Geometry check sheet. Reference: the model listing, model coordinates, mm. Coordinates: 2 decimals unless noted, no trailing zeros. Order: outer loops, then holes, each group sorted by start corner. A loop starts at its lowest first (then second) coordinate and runs counter-clockwise, first axis right, second up. Notation, with made-up numbers: (55.25, 61.5) -> (93.25, 61.5) arc R26 ccw to (93.25, 76.5) -> close; hole circle Ø11 at (32.5, -3.5). An arc over 180 degrees is marked (long way). Answer in a Markdown table with one row per item. Add a question column.
Autodesk Inventor part; units mm, degrees
ref_plane "YZ Plane" through (0, 0, 0) normal (1, 0, 0) x (0, 1, 0)
ref_plane "XZ Plane" through (0, 0, 0) normal (0, 1, 0) x (-1, 0, 0)
ref_plane "XY Plane" through (0, 0, 0) normal (0, 0, 1) x (1, 0, 0)
sketch "Sketch1" plane through (0, 0, 0) normal (0, 0, 1) x (1, 0, 0)
  line L0 (500, 50) -> (-500, 50)
  line L1 (-500, 50) -> (-500, -50)
  line L2 (-500, -50) -> (500, -50)
  line L3 (500, -50) -> (500, 50)
  line L4 (500, 50) -> (-500, -50) construction
  line L5 (-500, 50) -> (500, -50) construction
  point P0 (0, 0)
  dimension "d0" = 1000
  dimension "d1" = 100
sketch "Sketch2" plane through (0, 0, 0) normal (0, 0, 1) x (1, 0, 0)
  line L0 (400, 5) -> (450, 5)
  line L1 (400, -5) -> (450, -5)
  arc A0 (400, 5) -> (400, -5) centre (400, 0) ccw
  arc A1 (450, -5) -> (450, 5) centre (450, 0) ccw
  line L2 (-25, 5) -> (25, 5)
  line L3 (-25, -5) -> (25, -5)
  arc A2 (25, -5) -> (25, 5) centre (25, 0) ccw
  arc A3 (-25, 5) -> (-25, -5) centre (-25, 0) ccw
  line L4 (-450, 5) -> (-400, 5)
  line L5 (-450, -5) -> (-400, -5)
  arc A4 (-400, -5) -> (-400, 5) centre (-400, 0) ccw
  arc A5 (-450, 5) -> (-450, -5) centre (-450, 0) ccw
  point P0 (0, 0)
extrude "Extrusion1" add sketch "Sketch1" along normal blind 10
extrude "Extrusion2" cut sketch "Sketch2" along normal blind 10
properties part number "Sides"
(1) Go/stop test with a flat-tipped pin: P1, Ø8, axis at x = -221, y = -13, coming from the -Z side. Record where the tip stops, or that it passes through.
(2) Cross-section at B-B (z = 8.5). Enter the section's corners in (x, y), plus the area to 3 significant figures.
(3) Cross-section at A-A (x = 0.5). Enter the section's corners in (y, z).
(4) Scan lines: line 1 along X through (y, z) = (1, 9); line 2 along X through (y, z) = (3.5, 0.5); line 3 along Y through (x, z) = (-397, 8). Record each from-to range of solid material in increasing order.
Checks:
| question | item | result |
|---|---|---|
| 1 | P1 | z = 0 |
| 2 | outline | (-500, -50) -> (500, -50) -> (500, 50) -> (-500, 50) -> close; hole (-450, -5) -> (-400, -5) arc R5 ccw to (-400, 5) -> (-450, 5) arc R5 ccw to start; hole (-25, -5) -> (25, -5) arc R5 ccw to (25, 5) -> (-25, 5) arc R5 ccw to start; hole (400, -5) -> (450, -5) arc R5 ccw to (450, 5) -> (400, 5) arc R5 ccw to start |
| 2 | area | 98,300 mm² |
| 3 | outline | (-50, 0) -> (-5, 0) -> (-5, 10) -> (-50, 10) -> close; (5, 0) -> (50, 0) -> (50, 10) -> (5, 10) -> close |
| 4 | line 1 | -500 to -454.9, -395.1 to -29.9, 29.9 to 395.1, 454.9 to 500 |
| 4 | line 2 | -500 to -453.57, -396.43 to -28.57, 28.57 to 396.43, 453.57 to 500 |
| 4 | line 3 | -50 to -4, 4 to 50 |
